Model file for the job. Use its own axes, mm. A direction names the side the tool comes from. Coordinates: 2 decimals unless noted, no trailing zeros. Write each loop counter-clockwise with the first axis right and the second up, starting at its lowest first coordinate (ties: lowest second). Pieces come first, ordered by that corner, then holes. Notation, with made-up numbers: M 31,72 L 47,72 A26 cw 47,87 Z; hole C 13.5,24.25 d3. An arc over 180 degrees is marked long. Answer in a Markdown table with one row per item. Add a question column.
Autodesk Inventor part; units mm, degrees
ref_plane "pusher_XY" through (7, 0, 0) normal (1, 0, 0) x (0, 0, -1)
ref_plane "pusher_YZ" through (7, 0, 0) normal (0, 0, -1) x (0, 1, 0)
ref_plane "pusher_ZX" through (7, 0, 0) normal (0, 1, 0) x (1, 0, 0)
sketch "Sketch_1" plane through (0, 0, 0) normal (0, 0, 1) x (1, 0, 0)
  line L0 (12, 0) -> (0, 0)
  line L1 (0, 0) -> (0, 3)
  arc A0 (1, 4) -> (0, 3) centre (1, 3) ccw
  line L2 (1, 4) -> (7, 4)
  line L3 (7, 4) -> (7, 2.5)
  line L4 (7, 2.5) -> (3.5, 2.5)
  line L5 (3.5, 2.5) -> (2.5, 1.5)
  line L6 (2.5, 1.5) -> (2.5, 0)
  line L7 (2.5, 0) -> (0, 0)
revolve "Revolution1" add sketch "Sketch_1" angle 360 about axis through (12, 0, 0) along (1, 0, 0)
ref_plane "pusher_XY" through (7, 0, 0) normal (1, 0, 0) x (0, 0, -1)
ref_plane "pusher_YZ" through (7, 0, 0) normal (0, 0, -1) x (0, 1, 0)
ref_plane "pusher_ZX" through (7, 0, 0) normal (0, 1, 0) x (1, 0, 0)
properties part number "URLM8_p"
1) Flat gauge pins, fed straight in: pin 1 Ø2 at (x, z) = (2, 1) entering from -Y; pin 2 Ø3 at (x, z) = (5, 2) entering from +Y; pin 3 Ø2 at (y, z) = (1, -1) entering from +X; pin 4 Ø0.9 at (y, z) = (0, 0) entering from +X. Where does each tip first touch, or does it go through?
2) Slice it at C-C (x = 2.75). Give the cut face in (y, z).
3) Slice it at D-D (x = 1.25). Give the cut face in (y, z), then the cut area to 3 significant figures.
4) Slice it at A-A (y = 0). Give the cut face in (x, z), then the cut area to 3 significant figures.
5) Drill centre lines: probe 1 along Z at (x, y) = (4.35, 0); probe 2 along Z at (x, y) = (5.75, -1.75); probe 3 along Y at (x, z) = (6.25, 2). Where is each one in solid material? Low to high.
6) Two-plate mould, pull along Y, no slides. Class faces 3 (the face through (4.042, -0.867, -3.905)), 4 (the face through (0, 0, 0)), 5 (the face through (5.23, -0.54, 2.44)): released by +Y, released by -Y, zero draft, split by the parting line, or undercut.
7) Which spindle directions (+Z, -Z, +X, -X, +Y, -Y) get a long thin tool onto all of the face, cutting with end or side? Do faces 1 (the face through (2.5, 0, 0)), 2 (the face through (7, 2, 2)). Say none if no direction does.
Ans:
| question | item | result |
|---|---|---|
| 1 | pin 1 | stops at y = -4 |
| 1 | pin 2 | stops at y = 3.97 |
| 1 | pin 3 | stops at x = 3.41 |
| 1 | pin 4 | stops at x = 2.5 |
| 2 | outline | C 0,0 d8; hole C 0,0 d3.5 |
| 3 | outline | C 0,0 d8 |
| 3 | area | 50.3 mm2 |
| 4 | outline | M 0,-3 A1 ccw 1,-4 L 7,-4 L 7,-2.5 L 3.5,-2.5 L 2.5,-1.5 L 2.5,1.5 L 3.5,2.5 L 7,2.5 L 7,4 L 1,4 A1 ccw 0,3 Z |
| 4 | area | 34.1 mm2 |
| 5 | probe 1 | z = -4 to -2.5, 2.5 to 4 |
| 5 | probe 2 | z = -3.6 to -1.79, 1.79 to 3.6 |
| 5 | probe 3 | y = -3.46 to -1.5, 1.5 to 3.46 |
| 6 | face 3 | split by the parting line |
| 6 | face 4 | zero draft |
| 6 | face 5 | undercut |
| 7 | face 1 | +X |
| 7 | face 2 | +Z, -Z, +X, +Y, -Y |
